Read the model definition and answer for the solid it produces. Units are mm, in the model's axes. Face numbers are marked on the shaded views. A direction names the side the tool comes from. Coordinates: 2 decimals unless noted, no trailing zeros. Loops run counter-clockwise (first coordinate to the right, second up) from the corner with the lowest first, then second, coordinate; pieces in that order, holes last.
from build123d import *

# Parameters (mm, degrees)
SALIENTE_EXTRUIR1_DEPTH = 50.8
SALIENTE_EXTRUIR2_DEPTH = 9.525
SALIENTE_EXTRUIR3_DEPTH = 50.8
SALIENTE_EXTRUIR4_DEPTH = 9.525
CROQUIS5_W              = 19.05
CROQUIS5_H              = 9.525
CORTAR_EXTRUIR1_DEPTH   = 25


with BuildPart() as part:
    # Croquis1 → Saliente-Extruir1 (new body)
    with BuildSketch(Plane.XY):
        Polygon((0, 0), (0, 760), (-9.525, 760), (-9.525, 9.525), (-500, 9.525), (-500, 0), align=None)
    extrude(amount=SALIENTE_EXTRUIR1_DEPTH)

    # Croquis2 → Saliente-Extruir2 (add)
    with BuildSketch(Plane(origin=(0, 0, 0), x_dir=(-1, 0, 0), z_dir=(0, 0, -1))):
        Polygon((0, 760), (0, 0), (500, 0), (500, 50.8), (50.8, 50.8), (50.8, 760), align=None)
    extrude(amount=-SALIENTE_EXTRUIR2_DEPTH)

    # Croquis3 → Saliente-Extruir3 (add)
    with BuildSketch(Plane.XY.offset(9.525)):
        Polygon((-9.525, 280), (-115.591017178, 386.066017178), (-108.855825087, 392.801209269), (-9.525, 293.470384182), align=None)
        Polygon((-304.735424949, 9.525), (-318.205809131, 9.525), (-405.168921743, 96.488112613), (-398.433729653, 103.223304703), align=None)
    extrude(amount=SALIENTE_EXTRUIR3_DEPTH)

    # Croquis4 → Saliente-Extruir4 (add)
    with BuildSketch(Plane.XY.offset(9.525)):
        Polygon((-9.525, 280), (-115.591017178, 386.066017178), (-144.776849571, 356.880184785), (-9.525, 221.628335213), align=None)
        Polygon((-398.433729653, 103.223304703), (-304.735424949, 9.525), (-246.363760162, 9.525), (-369.247897259, 132.409137097), align=None)
    extrude(amount=SALIENTE_EXTRUIR4_DEPTH)

    # Croquis5 → Cortar-Extruir1 (cut)
    with BuildSketch(Plane(origin=(-250.828517178, 250.828517178, 0), x_dir=(0, 0, 1), z_dir=(-0.7071067811865419, 0.7071067811865532, 0))):
        with Locations((45.8, 196.017206641)):
            Rectangle(CROQUIS5_W, CROQUIS5_H)
        with Locations((50.8, -213.507793359)):
            Rectangle(CROQUIS5_W, CROQUIS5_H)
    extrude(amount=-CORTAR_EXTRUIR1_DEPTH, mode=Mode.SUBTRACT)


solid = part.part
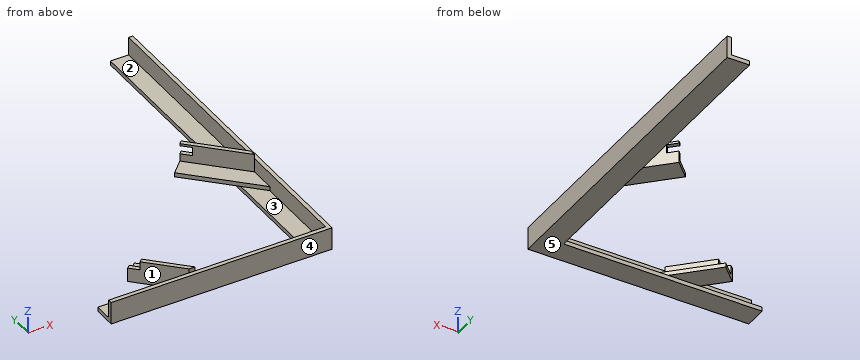
Q1. Straight lines are drawn through the part: probe 1 along Z at (x, y) = (-220, 38) (3 decimals); probe 2 along X at (y, z) = (491, 22.5) (3 decimals). For each, find the intervals that lie inside material, in ascending order.
Findings below:
probe 1: z = 0 to 9.525
probe 2: x = -9.525 to 0
Q2. Which of the six approach directions +Z, -Z, +X, -X, +Y, -Y give full straight-line access (tool end or side, diameter ignored) to the marked faces 1 and 2?
Findings below:
face 1: +Z, -X
face 2: +Z, +Y
Q3. Flat-ended cylindrical pins translate along their axes: pin 1 Ø3 at (x, z) = (-229, 6) entering from +Y; pin 2 Ø1.5 at (y, z) = (395.5, 30) entering from -X (3 decimals); pin 3 Ø12 at (x, z) = (-297.5, 36) entering from +Y (3 decimals). Find the tip coordinate at first contact, or state that the pin passes through.
Findings below:
pin 1: stops at y = 50.8
pin 2: stops at x = -9.525
pin 3: stops at y = 9.525
Q4. Determine the mould class of the marked faces 3, 4 and 5 for opening direction Y: +Y half, -Y half, draft (parallel to the pull), parting line (faces both ways), or undercut.
Findings below:
face 3: undercut
face 4: -Y half
face 5: draft
Q5. A cutting plane is placed at A-A (x = -184.5). Give the vertices of the cut face in (y, z) (3 decimals), then the cut area to 3 significant figures.
Findings below:
outline: (0, 0) - (50.8, 0) - (50.8, 9.525) - (9.525, 9.525) - (9.525, 50.8) - (0, 50.8) - close
area: 877 mm2
Q6. A cutting plane is placed at C-C (y = 516.5). Give the vertices of the cut face in (x, z) (3 decimals).
Findings below:
outline: (-50.8, 0) - (0, 0) - (0, 50.8) - (-9.525, 50.8) - (-9.525, 9.525) - (-50.8, 9.525) - close
Q7. A cutting plane is placed at B-B (y = 242). Give the vertices of the cut face in (x, z) (3 decimals).
Findings below:
outline: (-50.8, 0) - (0, 0) - (0, 50.8) - (-9.525, 50.8) - (-9.525, 19.05) - (-29.897, 19.05) - (-29.897, 9.525) - (-50.8, 9.525) - close
